from build123d import *

# Parameters (mm, degrees)
F5_W      = 26.67
F5_H      = 26.67
F6_DEPTH  = 31.75
F7_R      = 13.335
F9_DEPTH  = 15.875
F8_R      = 13.335
F10_DEPTH = 15.875
F12_R     = 7.3025
F14_DEPTH = 63.5
F11_R     = 8.9408
F15_DEPTH = 45.72
F13_R     = 7.3025
F16_DEPTH = 63.5
F18_D     = 2.794
F19_D     = 2.794
F20_DEPTH = 1.27
F21_DEPTH = 1.27


with BuildPart() as f6:
    # F5 (on offset) → F6 (new body)
    with BuildSketch(Plane.XZ.offset(15.875)):
        Rectangle(F5_W, F5_H)
    extrude(amount=-F6_DEPTH)

    # F7 (on offset) → F9 (join)
    with BuildSketch(Plane.XZ.offset(15.875)):
        Circle(F7_R)
    extrude(amount=F9_DEPTH)

    # F8 (on offset) → F10 (join)
    with BuildSketch(Plane.XZ.offset(-15.875)):
        Circle(F8_R)
    extrude(amount=-F10_DEPTH)

    # F12 (on offset) → F14 (cut)
    with BuildSketch(Plane.XZ.offset(31.75)):
        Circle(F12_R)
    extrude(amount=-F14_DEPTH, mode=Mode.SUBTRACT)

    # F11 (on offset) → F15 (cut)
    with BuildSketch(Plane.XZ.offset(31.75)):
        Circle(F11_R)
    extrude(amount=-F15_DEPTH, mode=Mode.SUBTRACT)

    # F13 (on offset) → F16 (cut)
    with BuildSketch(Plane.XZ.offset(-31.75)):
        Circle(F13_R)
    extrude(amount=F16_DEPTH, mode=Mode.SUBTRACT)

    # F18 (through all)
    with Locations(Plane(origin=(0, 0, -13.335), x_dir=(1, 0, 0), z_dir=(0, 0, -1))):
        with Locations((-11.303, -5.8039)):
            Hole(F18_D / 2)

    # F19 (through all)
    with Locations(Plane(origin=(0, 0, -13.335), x_dir=(1, 0, 0), z_dir=(0, 0, -1))):
        with Locations((-11.303, 5.8039)):
            Hole(F19_D / 2)

    # F20 (cut): a face of the model
    f20_faces = [f6.faces().sort_by_distance(p)[0] for p in [
        (0.166086667, 0, 13.335),
    ]]
    extrude(f20_faces, amount=-F20_DEPTH, mode=Mode.SUBTRACT)

    # F21 (cut): a face of the model
    f21_faces = [f6.faces().sort_by_distance(p)[0] for p in [
        (0.166086667, 0, -13.335),
    ]]
    extrude(f21_faces, amount=-F21_DEPTH, mode=Mode.SUBTRACT)


solid = f6.part
Geometry: final body of the model. Coordinates: model frame, mm. A direction names the side the tool comes from. Round coordinates to 2 decimals unless told otherwise and drop trailing zeros. Write each loop counter-clockwise with the first axis right and the second up, starting at its lowest first coordinate (ties: lowest second). Pieces come first, ordered by that corner, then holes. Notation, with made-up numbers: M -27.5,-16 L -17.5,-16 A34 ccw -17.5,23 Z; hole C 64.25,81 d8. An arc over 180 degrees is marked long. Write item = value, one per line.
Item 1: Section query C-C on y = 9.5. Return loops of the section in (x, z) (3 decimals), then the cut area to 3 significant figures.
Findings:
outline = M -13.335,-12.065 L 13.335,-12.065 L 13.335,12.065 L -13.335,12.065 Z; hole C 0,0 d17.882
area = 392 mm^2
Item 2: Section query B-B on x = -3.5. Return loops of the section in (y, z) (3 decimals).
Findings:
outline = M -31.75,-12.867 L -15.875,-12.867 L -15.875,-12.065 L 15.875,-12.065 L 15.875,-12.867 L 31.75,-12.867 L 31.75,-6.409 L 13.97,-6.409 L 13.97,-8.227 L -31.75,-8.227 Z; M -31.75,8.227 L 13.97,8.227 L 13.97,6.409 L 31.75,6.409 L 31.75,12.867 L 15.875,12.867 L 15.875,12.065 L -15.875,12.065 L -15.875,12.867 L -31.75,12.867 Z
Item 3: Access query for faces 1 (the face through (0, 0, -12.065)), 2 (the face through (-3, 13.97, -7)), 3 (the face through (-12, 15.875, 9)). Directions: +Z, -Z, +X, -X, +Y, -Y. A direction counts if a zero-diameter tool reaches every point of the face in a straight line with its end or side. Return the directions, or none.
Findings:
face_1 = -Z, +X, -X
face_2 = -Y
face_3 = +Z, -X, +Y
Item 4: Pull-direction query (Y, two-part tool) for faces 4 (the face through (0, -15.875, 13)), 5 (the face through (-11, 15.875, -9)), 6 (the face through (11, -15.875, -10)); classes: pulls with the +Y half, pulls with the -Y half, needs draft (parallel to the pull), parting line crosses it, or undercut.
Findings:
face_4 = undercut
face_5 = pulls with the +Y half
face_6 = pulls with the -Y half
Item 5: Pin query (flat end, axial travel): P1, Ø1, axis at x = 9.5, y = 23, coming from the +Z side; P2, Ø5, axis at x = -5.5, y = -9, coming from the +Z side (3 decimals); P3, Ø2, axis at y = -23, z = 10, coming from the -X side. Return the tip coordinate at first contact, or that it passes through.
Findings:
P1 = 9.84
P2 = 12.065
P3 = -9.84
Item 6: Material intervals for line 1 along Z through (x, y) = (0, 20.25) (1 decimal); line 2 along Y through (x, z) = (-10.5, -9) (3 decimals); line 3 along Y through (x, z) = (-12, 4.25), sorted ascending. Write a range as [from, to].
Findings:
line_1 = [-13.3, -7.3], [7.3, 13.3]
line_2 = [-15.875, -6.947], [-4.661, 4.661], [6.947, 15.875]
line_3 = [-31.75, -7.01], [-4.59, 4.59], [7.01, 31.75]
Item 7: Section query A-A on z = -1. Return loops of the section in (x, y) (3 decimals), then the cut area to 3 significant figures.
Findings:
outline = M -13.335,-15.875 L -13.297,-15.875 L -13.297,-31.75 L -8.885,-31.75 L -8.885,13.97 L -7.234,13.97 L -7.234,31.75 L -13.297,31.75 L -13.297,15.875 L -13.335,15.875 Z; M 7.234,13.97 L 8.885,13.97 L 8.885,-31.75 L 13.297,-31.75 L 13.297,-15.875 L 13.335,-15.875 L 13.335,15.875 L 13.297,15.875 L 13.297,31.75 L 7.234,31.75 Z; hole C -11.303,-5.804 d2.794; hole C -11.303,5.804 d2.794
area = 609 mm^2
